Source: CAD feature listing. Evaluate the final solid. Frame: model axes, mm. Round coordinates to 2 decimals unless told otherwise and drop trailing zeros. Loops run counter-clockwise (first coordinate to the right, second up) from the corner with the lowest first, then second, coordinate; pieces in that order, holes last. Notation, with made-up numbers: M 5,69.25 L 16,69.25 A15 ccw 16,98.25 Z; hole C 34.5,89 d1. An arc over 180 degrees is marked long. One line per item, written item: value.
from build123d import *

# Parameters (mm, degrees)
F1_W     = 101.595435
F1_H     = 76.268525
F1_R     = 25.693818
F2_DEPTH = 25.4


with BuildPart() as f2:
    # F1 (on face) → F2 (new body)
    with BuildSketch(Plane.XZ):
        with Locations((-4.892697, 9.497589)):
            Rectangle(F1_W, F1_H)
        with Locations((-5.900017, 7.051241)):
            Circle(F1_R, mode=Mode.SUBTRACT)
    extrude(amount=F2_DEPTH)


solid = f2.part
1. Ray query, line 1 (Z direction, x = -28, y = -22); line 2 (X direction, y = -15, z = 16); line 3 (Z direction, x = -20, y = -11.25). Return the intervals inside material, ascending. Write a range as [from, to].
Report:
line 1: z = [-28.64, -6.05], [20.16, 47.63]
line 2: x = [-55.69, -29.99], [18.19, 45.91]
line 3: z = [-28.64, -14.43], [28.53, 47.63]
2. Section query A-A (z = 18.5). Return the cut outline in (x, y), and give its area (3 significant figures).
Report:
outline: M -55.69,-25.4 L -28.9,-25.4 L -28.9,0 L -55.69,0 Z; M 17.1,-25.4 L 45.91,-25.4 L 45.91,0 L 17.1,0 Z
area: 1,410 mm2
3. Section query B-B (x = -27.5). Return the cut outline in (y, z), and give its area (3 significant figures).
Report:
outline: M -25.4,-28.64 L 0,-28.64 L 0,-6.86 L -25.4,-6.86 Z; M -25.4,20.97 L 0,20.97 L 0,47.63 L -25.4,47.63 Z
area: 1,230 mm2
4. Section query C-C (y = -15.5). Return the cut outline in (x, z).
Report:
outline: M -55.69,-28.64 L 45.91,-28.64 L 45.91,47.63 L -55.69,47.63 Z; hole C -5.9,7.05 d51.39
5. Pull-direction query (Z, two-part tool) for faces 1 (the face through (-6, 0, 35)), 2 (the face through (-11.47, -12.52, -18.03)), 3 (the face through (-6, -13, -28.637)); classes: released by +Z, released by -Z, zero draft, split by the parting line, or undercut.
Report:
face 1: zero draft
face 2: undercut
face 3: released by -Z
